Part print with two shaded views. Sizes in mm from the minimum x, y, z corner. A direction names the side the tool comes from. Round coordinates to 2 decimals unless told otherwise and drop trailing zeros. Loops run counter-clockwise (first coordinate to the right, second up) from the corner with the lowest first, then second, coordinate; pieces in that order, holes last.
(1) Cut at C-C on y = 113. List the corners of the cut face in (x, z), then the cut area to 3 significant figures.
(2) Flat gauge pins, fed straight in: pin 1 (12 mm diameter, centred on x = 68, z = 55, fed in from -Y); pin 2 (14.5 mm diameter, centred on x = 154, z = 49.5, fed in from +Y) (3 decimals); pin 3 (10 mm diameter, centred on x = 62, y = 111, fed in from -Z); pin 4 (6 mm diameter, centred on y = 87, z = 91, fed in from -X). Where does each tip first touch, or does it go through?
(3) Mould opens along Y. For the marked faces 1, 2, 3 and 4 say: +Y half, -Y half, draft (parallel to the pull), parting line (faces both ways), or undercut.
(4) Tool access for the marked faces 5, 6, 7, 8 and 9: list every direction of +Z, -Z, +X, -X, +Y, -Y with a clear straight run to the whole face (end or side of a thin tool).
(5) Probe probe 1 along Y at (x, z) = (167, 68) (1 decimal); probe 2 along X at (y, z) = (47.5, 53); probe 3 along Z at (x, y) = (52, 116). List the from-to ranges inside material, lowest first.
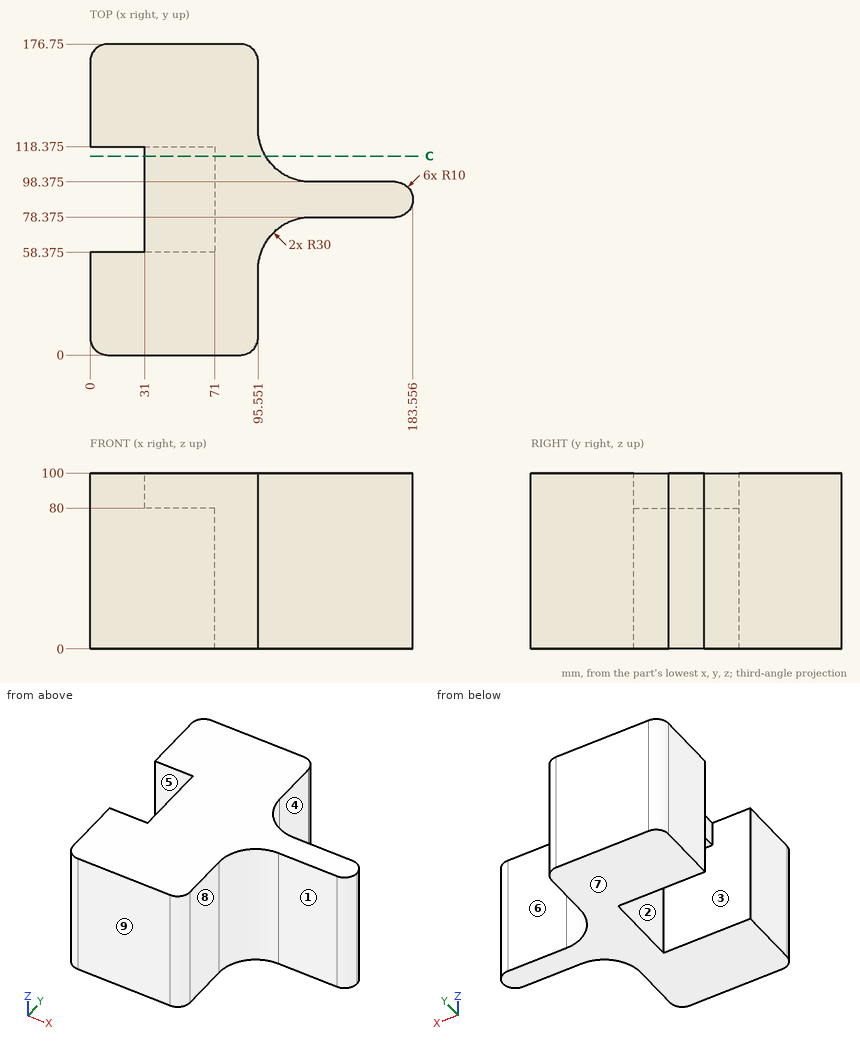
Final values:
1. outline: (31, 80) - (71, 80) - (71, 0) - (99.79, 0) - (99.79, 100) - (31, 100) - close
1. area: 3,680 mm2
2. pin 1: stops at y = 0
2. pin 2: stops at y = 98.375
2. pin 3: stops at z = 80
2. pin 4: stops at x = 31
3. face 1: -Y half
3. face 2: undercut
3. face 3: undercut
3. face 4: draft
4. face 5: -Z, -X
4. face 6: +Z, -Z, +X, +Y
4. face 7: -Z, +X, -X, +Y, -Y
4. face 8: +Z, -Z, +X, -Y
4. face 9: +Z, -Z, +X, -X, -Y
5. probe 1: y = 78.4 to 98.4
5. probe 2: x = 0 to 95.55
5. probe 3: z = 80 to 100
